Source: CAD feature listing. Evaluate the final solid. Frame: model axes, mm. Face numbers are marked on the shaded views. A direction names the side the tool comes from. Give positions to 0.01 mm unless a question says otherwise; leave off trailing zeros. Write each loop counter-clockwise with the first axis right and the second up, starting at its lowest first coordinate (ties: lowest second). Pieces come first, ordered by that corner, then holes. Notation, with made-up numbers: (-30, 28) - (-14, 28) arc R21 ccw to (-14, 37) - close; hole circle Ø1 at (63.25, -31). An arc over 180 degrees is marked (long way). Answer as a JSON object with one key per item and string values. Group by question number.
from build123d import *

# Parameters (mm, degrees)
F1_DEPTH = 63.5
F0_W     = 25.4
F0_H     = 19.05
F2_DEPTH = 25.4
F3_DEPTH = 15.875
F5_R     = 6.35


# Not quite as in the source:
# - a feature names something its author has since deleted; it is built from what else it names


with BuildPart() as f1:
    # F0 (on Front) → F1 (new body, symmetric)
    with BuildSketch(Plane.XZ):
        Polygon((41.275, -9.525), (41.275, 9.525), (22.225, 9.525), (-41.275, 9.525), (-41.275, -9.525), align=None)
    extrude(amount=F1_DEPTH, both=True)

    # F0 (on Front) → F2 (join, symmetric)
    with BuildSketch(Plane.XZ):
        with BuildLine():
            Line((22.225, 9.525), (41.275, 9.525))
            Line((41.275, 9.525), (41.275, 27.0002))
            ThreePointArc((41.275, 27.0002), (45.9246798487, 38.2255201513), (57.15, 42.8752))
            Line((57.15, 42.8752), (60.325, 42.8752))
            Line((60.325, 42.8752), (60.325, 61.9252))
            Line((60.325, 61.9252), (57.15, 61.9252))
            add(Edge.make_bspline(
                [(54.6259105013, 61.8338704526), (55.4670032291, 61.8648637063), (56.3085016145, 61.8950318532), (57.15, 61.9252)],
                knots=[0.9787843068, 0.9787843068, 0.9787843068, 0.9787843068, 1, 1, 1, 1], degree=3))
            ThreePointArc((54.6259105013, 61.8338704526), (31.5774614993, 50.7867697323), (22.225, 27.0002))
            Line((22.225, 27.0002), (22.225, 9.525))
        make_face()
        with Locations((73.025, 52.4002)):
            Rectangle(F0_W, F0_H)
    extrude(amount=F2_DEPTH, both=True)

    # F0 (on Front) → F3 (join)
    with BuildSketch(Plane.XZ):
        with BuildLine():
            Line((-41.275, 9.525), (22.225, 9.525))
            Line((22.225, 9.525), (22.225, 27.0002))
            ThreePointArc((22.225, 27.0002), (31.5774614993, 50.7867697323), (54.6259105013, 61.8338704526))
            add(Edge.make_bspline(
                [(-41.275, 9.525), (-31.2937791868, 20.1864348925), (-12.273821172, 40.5025913853), (17.5953077761, 60.105451895), (42.3186244489, 61.380361789), (54.6259105013, 61.8338704526)],
                knots=[0, 0, 0, 0, 0.3507319306, 0.6683457584, 0.9787843068, 0.9787843068, 0.9787843068, 0.9787843068], degree=3))
        make_face()
    extrude(amount=F3_DEPTH)

    # F0 (on Front) → F4 (revolve)
    with BuildSketch(Plane.XZ):
        Polygon((85.725, 61.9252), (85.725, 42.8752), (85.725, 38.1), (111.125, 38.1), (111.125, 66.675), (85.725, 66.675), align=None)
    revolve(axis=Axis((85.725, 0, 52.3875), (0, 0, -1)))

    # F5
    f5_edges = [f1.edges().sort_by_distance(p)[0] for p in [
        (-41.275, -63.5, 0),
        (-41.275, 63.5, 0),
        (41.275, 63.5, 0),
        (41.275, -63.5, 0),
    ]]
    fillet(f5_edges, radius=F5_R)


solid = f1.part
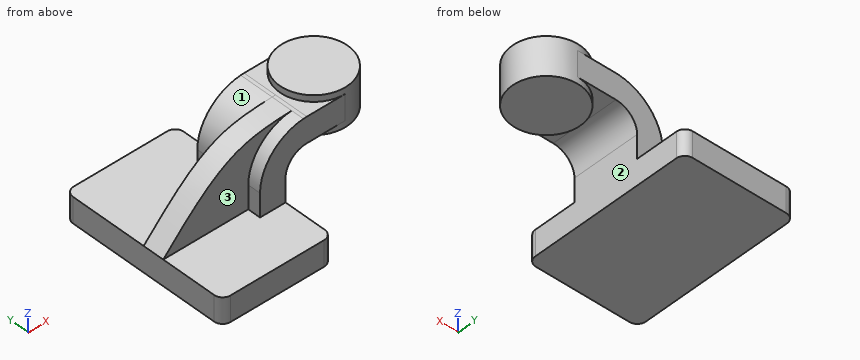
Q1. Section C-C on x = 84. Return the cut outline in (y, z) (3 decimals).
Q2. Ray query, probe 1 along X at (y, z) = (-5, 5) (3 decimals); probe 2 along Z at (x, y) = (-4, 54.5) (3 decimals); probe 3 along X at (y, z) = (19.5, 14.5) (3 decimals). Return the intervals inside material, ascending. Write a range as [from, to].
Q3. First-contact query: pin 1 Ø19 at (x, y) = (-0.5, 35) entering from +Z (3 decimals); pin 2 Ø3 at (y, z) = (-9.5, 48) entering from +X; pin 3 Ø1 at (x, y) = (50, -9) entering from -Z. Flat tips, straight axial feed; report the tip coordinate or a pass-through.
Q4. Reachability of the marked faces 1, 2 and 3 from +Z, -Z, +X, -X, +Y, -Y: full face, straight path, thin tool, end or side. Return the list, or none.
Q5. Section B-B on y = -40. Return the cut outline in (x, z) (3 decimals).
Q6. Section D-D on x = 100. Return the cut outline in (y, z) (3 decimals), then the cut area to 3 significant figures.
Q7. Section A-A on z = 3. Return the cut outline in (x, y) (3 decimals).
Taken from the geometry:
{
 "1": {"outline": "(-25.4, 42.875) - (-25.341, 42.875) - (-25.341, 38.1) - (25.341, 38.1) - (25.341, 42.875) - (25.4, 42.875) - (25.4, 61.925) - (25.341, 61.925) - (25.341, 66.675) - (-25.341, 66.675) - (-25.341, 61.925) - (-25.4, 61.925) - close"},
 "2": {"probe 1": "x = [-41.275, 41.275]", "probe 2": "z = [-9.525, 9.525]", "probe 3": "x = [22.225, 41.275]"},
 "3": {"pin 1": "stops at z = 9.525", "pin 2": "stops at x = 109.83", "pin 3": "stops at z = 40.91"},
 "4": {"face 1": "+Z, -X, +Y", "face 2": "-Z, +X, +Y, -Y", "face 3": "+Z, -X, -Y"},
 "5": {"outline": "(-41.275, -9.525) - (41.275, -9.525) - (41.275, 9.525) - (-41.275, 9.525) - close"},
 "6": {"outline": "(-21.009, 38.1) - (21.009, 38.1) - (21.009, 66.675) - (-21.009, 66.675) - close", "area": "1,200 mm²"},
 "7": {"outline": "(-41.275, -57.15) arc R6.35 ccw to (-34.925, -63.5) - (34.925, -63.5) arc R6.35 ccw to (41.275, -57.15) - (41.275, 57.15) arc R6.35 ccw to (34.925, 63.5) - (-34.925, 63.5) arc R6.35 ccw to (-41.275, 57.15) - close"}
}
